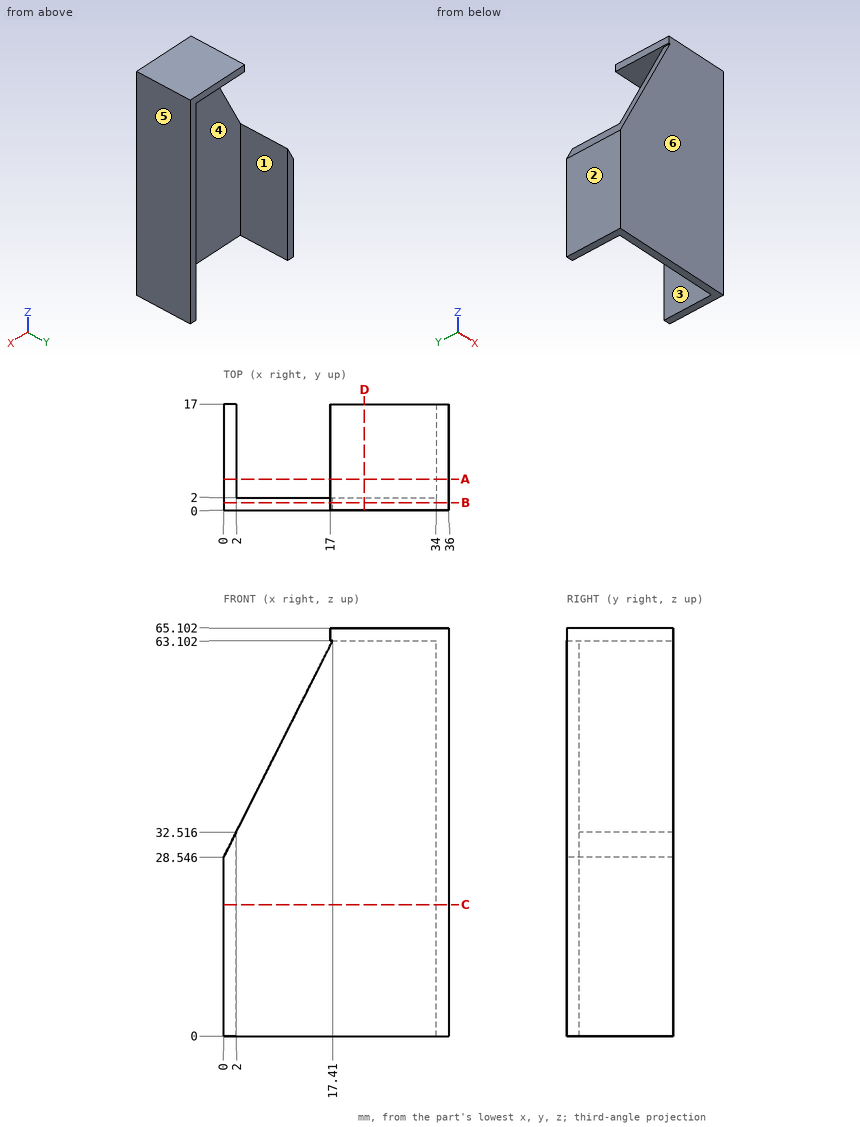
Input: dimensioned drawing with shaded views. Units: mm. Origin: part minimum x, y, z. A direction names the side the tool comes from. Round coordinates to 2 decimals unless told otherwise and drop trailing zeros. Write each loop counter-clockwise with the first axis right and the second up, starting at its lowest first coordinate (ties: lowest second). Pieces come first, ordered by that corner, then holes. Notation, with made-up numbers: (-37.5, 1.5) -> (11.5, 1.5) arc R22 ccw to (11.5, 7.5) -> close; hole circle Ø1 at (-24.75, 47.25). An arc over 180 degrees is marked (long way). Use CSV: the item, a comma, the result in double quotes. Start each with the question number.
Q1. Line query: L1, parallel to X at y = 13.75, z = 23.5; L2, parallel to X at y = 7.25, z = 40; L3, parallel to Z at x = 27.5, y = 3.75. Output: solid intervals per line, ascending.
Q2. First-contact query: pin 1 Ø9.5 at (x, z) = (15, 27) entering from +Y; pin 2 Ø1 at (y, z) = (9, 64) entering from -X; pin 3 Ø5 at (x, y) = (23, 7.5) entering from -Z. Flat tips, straight axial feed; report the tip coordinate or a pass-through.
Q3. Section C-C (z = 21). Return loops of the section in (x, y), plus the area to 3 significant figures.
Q4. Section D-D (x = 22.5). Return loops of the section in (y, z).
Q5. Section B-B (y = 1.25). Return loops of the section in (x, z), plus the area to 3 significant figures.
Q6. Section A-A (y = 5). Return loops of the section in (x, z), plus the area to 3 significant figures.
Q7. Reachability of the marked faces 1 and 2 from +Z, -Z, +X, -X, +Y, -Y: full face, straight path, thin tool, end or side. Return the list, or none.
Q8. Pull-direction query (X, two-part tool) for the marked faces 3, 4, 5 and 6; classes: pulls with the +X half, pulls with the -X half, needs draft (parallel to the pull), parting line crosses it, or undercut.
Result sheet:
1,L1,"0 to 2, 34 to 36"
1,L2,"34 to 36"
1,L3,"63.1 to 65.1"
2,pin 1,"y = 2"
2,pin 2,"x = 17"
2,pin 3,"z = 63.1"
3,outline,"(0, 0) -> (36, 0) -> (36, 17) -> (34, 17) -> (34, 2) -> (2, 2) -> (2, 17) -> (0, 17) -> close"
3,area,"132 mm²"
4,outline,"(0, 0) -> (2, 0) -> (2, 63.1) -> (17, 63.1) -> (17, 65.1) -> (0, 65.1) -> close"
5,outline,"(0, 0) -> (36, 0) -> (36, 65.1) -> (17, 65.1) -> (17, 63.1) -> (17.41, 63.1) -> (0, 28.55) -> close"
5,area,"2,010 mm²"
6,outline,"(0, 0) -> (2, 0) -> (2, 32.52) -> (0, 28.55) -> close; (17, 63.1) -> (34, 63.1) -> (34, 0) -> (36, 0) -> (36, 65.1) -> (17, 65.1) -> close"
6,area,"225 mm²"
7,face 1,"+Z, -Z, +Y"
7,face 2,"+Z, -Z, -X, +Y, -Y"
8,face 3,"undercut"
8,face 4,"undercut"
8,face 5,"pulls with the +X half"
8,face 6,"needs draft"
